```python
from build123d import *

# Parameters (mm, degrees)
F1_DEPTH = 25.4
F3_DEPTH = 19.05
F5_DEPTH = 6.35
F6_R     = 3.175
F7_DEPTH = 67.7343333333


with BuildPart() as f1:
    # F0 (on Front) → F1 (new body, symmetric)
    with BuildSketch(Plane.XZ):
        Polygon((38.1, 63.5), (0, 63.5), (0, 25.4), (25.4, 0), (76.2, 0), (76.2, 50.8), align=None)
    extrude(amount=F1_DEPTH, both=True)

    # F2 (on Front) → F3 (join)
    with BuildSketch(Plane.XZ):
        Polygon((63.5, 67.7333333333), (63.5, 55.0333333333), (76.2, 50.8), (76.2, 0), (114.3, 0), (114.3, 25.4), (101.6, 29.6333333333), (101.6, 67.7333333333), align=None)
    extrude(amount=-F3_DEPTH)

    # F4 (on face) → F5 (join)
    with BuildSketch(Plane(origin=(0, 19.05, 0), x_dir=(-1, 0, 0), z_dir=(0, 1, 0))):
        Polygon((-101.6, 29.6333333333), (-114.3, 25.4), (-114.3, 0), (-76.2, 0), (-76.2, 38.1), align=None)
    extrude(amount=F5_DEPTH)

    # F6 (on face) → F7 (cut, through all)
    with BuildSketch(Plane.XY.offset(67.7333333333)):
        with Locations((73.025, 9.525)):
            Circle(F6_R)
        with Locations((92.075, 9.525)):
            Circle(F6_R)
    extrude(amount=-F7_DEPTH, mode=Mode.SUBTRACT)


solid = f1.part
```
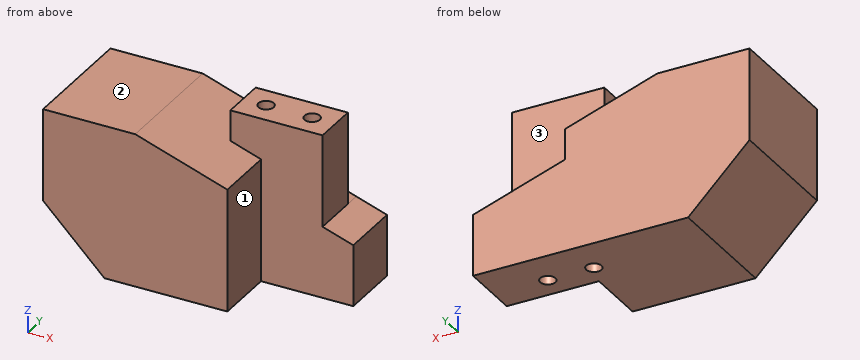
Could you check a few things on this model? Use its own coordinates, in mm. Face numbers are marked on the shaded views. A direction names the side the tool comes from. Round coordinates to 2 decimals unless told otherwise and drop trailing zeros. Order: outer loops, then holes, each group sorted by start corner. A loop starts at its lowest first (then second) coordinate and runs counter-clockwise, first axis right, second up. Notation, with made-up numbers: M 35,31.25 L 93,31.25 A19 cw 93,39.25 Z; hole C 8,-27.5 d7. An arc over 180 degrees is marked long. One line per question, with ' | ' between items. Start each with the question number.
(1) For P1, Ø5, axis at x = 79.5, z = 47.5, coming from the +Y side; P2, Ø3, axis at y = 12, z = 36, coming from the +X side; P3, Ø8, axis at x = 65, y = -5, coming from the +Z side, each with a flat end and sliding along its axis, tell me the tip position at first contact or that it passes through.
(2) Suppose I cut it at A-A on z = 57. List the corners of the cut face in (x, y) for me (3 decimals).
(3) Suppose I cut it at B-B on x = 75. List the corners of the cut face in (y, z) for me, then the cut area to 3 significant figures.
(4) Suppose I cut it at C-C on y = 3. List the corners of the cut face in (x, z) for me.
(5) Suppose I cut it at D-D on z = 22. List the corners of the cut face in (x, y) for me (3 decimals).
(6) Please list where these lines run through material, in increasing order: line 1 along X through (y, z) = (-18.5, 46); line 2 along X through (y, z) = (18.5, 49); line 3 along Z through (x, y) = (34, -4.5).
(7) For the marked faces 1, 2 and 3, which set-ups out of +Z, -Z, +X, -X, +Y, -Y let a thin tool reach every point of the face, with its end or its side?
Geometry results:
1) P1: y = 19.05 | P2: x = 101.6 | P3: z = 55.87
2) outline: M 0,-25.4 L 57.6,-25.4 L 57.6,25.4 L 0,25.4 Z; M 63.5,0 L 101.6,0 L 101.6,19.05 L 63.5,19.05 Z; hole C 73.025,9.525 d6.35; hole C 92.075,9.525 d6.35
3) outline: M -25.4,0 L 7.04,0 L 7.04,67.73 L 0,67.73 L 0,51.2 L -25.4,51.2 Z; M 12.01,0 L 25.4,0 L 25.4,51.2 L 19.05,51.2 L 19.05,67.73 L 12.01,67.73 Z | area: 2,580 mm²
4) outline: M 0,25.4 L 25.4,0 L 114.3,0 L 114.3,25.4 L 101.6,29.63 L 101.6,67.73 L 63.5,67.73 L 63.5,55.03 L 38.1,63.5 L 0,63.5 Z
5) outline: M 3.4,-25.4 L 76.2,-25.4 L 76.2,0 L 114.3,0 L 114.3,25.4 L 3.4,25.4 Z; hole C 73.025,9.525 d6.35; hole C 92.075,9.525 d6.35
6) line 1: 0 to 76.2 | line 2: 0 to 101.6 | line 3: 0 to 63.5
7) face 1: +Z, -Z, +X, -Y | face 2: +Z, -X, +Y, -Y | face 3: +Z, +X, +Y
